Verification items for the finished model (mm, model axes). A direction names the side the tool comes from. Round coordinates to 2 decimals unless told otherwise and drop trailing zeros. Write each loop counter-clockwise with the first axis right and the second up, starting at its lowest first coordinate (ties: lowest second). Pieces come first, ordered by that corner, then holes. Notation, with made-up numbers: (-17, 40.5) - (-4, 40.5) arc R26 ccw to (-4, 72.5) - close; hole circle Ø11 at (41.5, -9.5). An arc over 180 degrees is marked (long way). Answer as a JSON object with one key per item and string values. Group by question number.
1) Section check C-C (x = -11). Enter the section's corners in (y, z), then the cut area to 3 significant figures.
2) Go/stop test with flat-tipped pins: pin 1 Ø2 at (x, z) = (4.93, -18.4) entering from +Y; pin 2 Ø10 at (x, y) = (-20.5, 12) entering from -Z; pin 3 Ø6 at (x, y) = (21.5, 18.5) entering from +Z. Record where each tip stops, or that it passes through.
3) Section check A-A (z = 0). Enter the section's corners in (x, y) (3 decimals), then the cut area to 3 significant figures.
4) Mould release check, pull along X, two halves, no side actions. Record for faces 1 (the cylindrical face through (5.5, -32.7, 28.4)), 2 (the cylindrical face through (-19.752, 35.142, -4.871)), 3 (the flat face through (0, -38.1, 0)): +X half, -X half, draft (parallel to the pull), parting line (faces both ways), or undercut.
5) Thickness scan on line 1 (Y direction, x = 21.5, z = 3.5); line 2 (Z direction, x = 10.5, y = -27); line 3 (X direction, y = -29, z = 6). Record the ranges inside material, lowest first.
6) Set-up check for faces 4 (the cylindrical face through (1.93, 47.76, 2.52)), 5 (the flat face through (0, -33, 30.075)): record each of +Z, -Z, +X, -X, +Y, -Y from which the full face is reachable in a straight line by a thin tool's end or side.
7) Section check D-D (y = 17). Enter the section's corners in (x, z) (3 decimals), then the cut area to 3 significant figures.
8) Section check B-B (y = 40). Enter the section's corners in (x, z) (3 decimals), then the cut area to 3 significant figures.
```python
from build123d import *

# Parameters (mm, degrees)
SKETCH2_R           = 5.5
BOSS_EXTRUDE1_DEPTH = 1.5
CIRPATTERN1_COUNT   = 4
FILLET2_SIZE        = 1.5


with BuildPart() as part:
    # Sketch1 → Revolve1 (revolve)
    with BuildSketch(Plane.XY, mode=Mode.PRIVATE) as revolve1_sk:
        Polygon((0, 38.1), (0, -38.1), (28.575, -38.1), (28.575, 38.1), (3.175, 38.1), (3.175, 57.15), (0, 57.15), align=None)
    revolve(revolve1_sk.sketch.rotate(Axis((0, 0, 0), (0, 1, 0)), 90), axis=Axis((0, 0, 0), (0, 1, 0)))

    # Sketch2 → Boss-Extrude1 (add, symmetric)
    with BuildSketch(Plane.XY.offset(28.575)):
        with Locations(Location((0, -32.6, 0), (0, 0, 270))):
            Circle(SKETCH2_R)
    extrude(amount=BOSS_EXTRUDE1_DEPTH, both=True)

    # Sketch5 → #6-32 Tapped Hole1 (revolve, cut)
    with BuildSketch(Plane(origin=(4.930502809, 38.1, -18.400886991), x_dir=(0, 0, 1), z_dir=(1, 0, 0))):
        Polygon((0, 0), (0, 6.81269403), (1.35255, 6), (1.35255, 0), align=None)
    f_6_32_tapped_hole1 = revolve(axis=Axis((4.930502809, 44.45, -18.400886991), (0, -1, 0)), mode=Mode.SUBTRACT)

    # CirPattern1: #6-32 Tapped Hole1 ×4 about axis
    cirpattern1_axis = Axis((0, 0, 0), (0, 1, 0))
    for i in range(1, CIRPATTERN1_COUNT):
        add(f_6_32_tapped_hole1.rotate(cirpattern1_axis, i * 360 / CIRPATTERN1_COUNT), mode=Mode.SUBTRACT)

    # Fillet2
    # a fillet whose section is not a circle: 1.5 mm, written as the material it takes off along each edge
    with BuildSketch(Plane(origin=(0, -32.6, 30.075), x_dir=(0, -1, 0), z_dir=(-1, 0, 0))) as fillet2_piece_1_section:
        with BuildLine():
            Bezier((5.5, -FILLET2_SIZE), (5.5, 0), (5.5 - FILLET2_SIZE, 0), weights=[1, 0.333333333, 1])
            Line((5.5 - FILLET2_SIZE, 0), (5.5, 0))
            Line((5.5, 0), (5.5, -FILLET2_SIZE))
        make_face()
    fillet2_piece_1 = revolve(axis=Axis((0, -32.6, 30.075), (0, 0, 1)), mode=Mode.PRIVATE)
    fillet2_piece_1 = fillet2_piece_1 - Plane(origin=(0, -32.6, 0), x_dir=(0, 0, -1), z_dir=(0, 1, 0)) * Cylinder(28.575, 22, mode=Mode.PRIVATE)
    add(fillet2_piece_1, mode=Mode.SUBTRACT)


solid = part.part
```
Returned:
{
 "1": {"outline": "(-38.1, -26.37) - (38.1, -26.37) - (38.1, 26.37) - (-38.1, 26.37) - close", "area": "4,020 mm2"},
 "2": {"pin 1": "y = 31.89", "pin 2": "z = -24.01", "pin 3": "z = 21.78"},
 "3": {"outline": "(-28.575, -38.1) - (28.575, -38.1) - (28.575, 38.1) - (3.175, 38.1) - (3.175, 57.15) - (-3.175, 57.15) - (-3.175, 38.1) - (-28.575, 38.1) - close", "area": "4,480 mm2"},
 "4": {"face 1": "+X half", "face 2": "undercut", "face 3": "draft"},
 "5": {"line 1": "-38.1 to 38.1", "line 2": "-26.58 to 26.58", "line 3": "-27.94 to 27.94"},
 "6": {"face 4": "+Y", "face 5": "+Z, +X, -X, +Y, -Y"},
 "7": {"outline": "circle Ø57.15 at (0, 0)", "area": "2,570 mm2"},
 "8": {"outline": "circle Ø6.35 at (0, 0)", "area": "31.7 mm2"}
}
